CAD build for the part. Positions are in the model's coordinates, mm. Give positions to 0.01 mm unless a question says otherwise; leave off trailing zeros. Loops run counter-clockwise (first coordinate to the right, second up) from the corner with the lowest first, then second, coordinate; pieces in that order, holes last. Notation, with made-up numbers: M -16,70.5 L 43,70.5 A11 cw 43,77.5 Z; hole C -7,40 d4. An arc over 180 degrees is marked long. Answer as CSV lines item,"result".
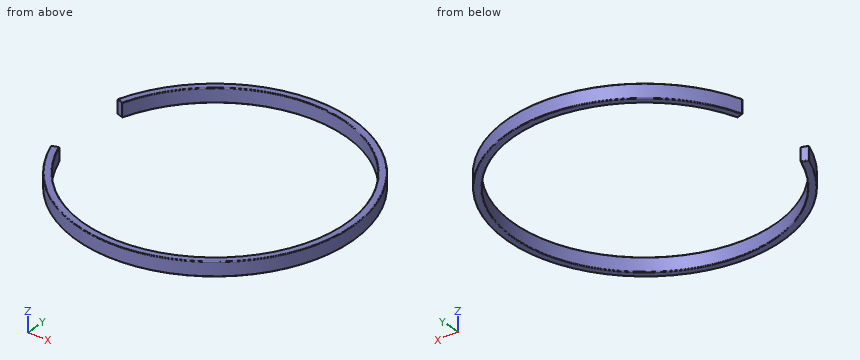
from build123d import *

# Parameters (mm, degrees)
F1_DEPTH = 1.016
F2_R     = 0.0508


with BuildPart() as f1:
    # F0 (on Top) → F1 (new body)
    with BuildSketch(Plane.XY):
        with BuildLine():
            Line((-8.880662, -3.036066), (-9.361347, -3.2004))
            ThreePointArc((-9.361347, -3.2004), (9.8933, 0), (-9.361347, 3.2004))
            Line((-9.361347, 3.2004), (-8.880662, 3.036066))
            ThreePointArc((-8.880662, 3.036066), (9.3853, 0), (-8.880662, -3.036066))
        make_face()
    extrude(amount=F1_DEPTH)

    # F2
    f2_edges = [f1.edges().sort_by_distance(p)[0] for p in [
        (9.3853, 0, 1.016),
        (9.8933, 0, 1.016),
        (9.8933, 0, 0),
        (9.3853, 0, 0),
        (-8.880662, -3.036066, 0.508),
        (-8.880662, 3.036066, 0.508),
        (-9.361347, 3.2004, 0.508),
        (-9.121005, 3.118233, 0),
        (-9.121005, 3.118233, 1.016),
        (-9.121005, -3.118233, 0),
        (-9.361347, -3.2004, 0.508),
        (-9.121005, -3.118233, 1.016),
    ]]
    fillet(f2_edges, radius=F2_R)


solid = f1.part
1) Flat gauge pin, fed straight in: pin 1 (2 mm diameter, centred on x = -6, y = 5.5, fed in from +Z). Where does the tip first touch, or does it go through?
Answer below:
pin 1,"passes through"
2) Band-saw the part on B-B on y = 0. Give the cut face in (x, z).
Answer below:
outline,"M 9.39,0.05 A0.05 ccw 9.44,0 L 9.84,0 A0.05 ccw 9.89,0.05 L 9.89,0.97 A0.05 ccw 9.84,1.02 L 9.44,1.02 A0.05 ccw 9.39,0.97 Z"
3) Drill centre lines: line 1 (Y direction, x = 0, z = 0.7); line 2 (Y direction, x = 1.25, z = 0.7); line 3 (X direction, y = 6, z = 0.35). Where is each one in solid material? Low to high. Write a range as from..to.
Answer below:
line 1,"y = -9.89..-9.39, 9.39..9.89"
line 2,"y = -9.81..-9.3, 9.3..9.81"
line 3,"x = -7.87..-7.22, 7.22..7.87"
4) Band-saw the part on A-A on z = 0.6. Give the cut face in (x, y), and give its area (3 significant figures).
Answer below:
outline,"M -9.34,-3.25 A9.89 ccw long -9.34,3.25 A0.05 ccw -9.31,3.18 L -8.93,3.05 A0.05 ccw -8.86,3.08 A9.39 cw long -8.86,-3.08 A0.05 ccw -8.93,-3.05 L -9.31,-3.18 A0.05 ccw Z"
area,"27.5 mm^2"
